Geometry: final body of the model. Coordinates: model frame, mm. Give positions to 0.01 mm unless a question says otherwise; leave off trailing zeros. Write each loop counter-clockwise with the first axis right and the second up, starting at its lowest first coordinate (ties: lowest second). Pieces come first, ordered by that corner, then holes.
```python
from build123d import *

# Parameters (mm, degrees)
SKIZZE2_W                       = 65
SKIZZE2_H                       = 12
AUFSATZ_LINEAR_AUSTRAGEN1_DEPTH = 4
SKIZZE3_R                       = 1.7
SCHNITT_LINEAR_AUSTRAGEN1_DEPTH = 70.241173381
SKIZZE4_R                       = 3.25
SCHNITT_LINEAR_AUSTRAGEN2_DEPTH = 3.2
VERRUNDUNG3_R                   = 1.2


with BuildPart() as part:
    # Skizze2 → Aufsatz-Linear austragen1 (new body)
    with BuildSketch(Plane.XY.offset(18)):
        with Locations((34.289745228, 11.817688499)):
            Rectangle(SKIZZE2_W, SKIZZE2_H)
    extrude(amount=AUFSATZ_LINEAR_AUSTRAGEN1_DEPTH)

    # Skizze3 → Schnitt-Linear austragen1 (cut, through all)
    with BuildSketch(Plane.XY.offset(22)):
        with Locations((21.789745228, 11.817688499)):
            Circle(SKIZZE3_R)
        with Locations((46.789745228, 11.817688499)):
            Circle(SKIZZE3_R)
    extrude(amount=-SCHNITT_LINEAR_AUSTRAGEN1_DEPTH, mode=Mode.SUBTRACT)

    # Skizze4 → Schnitt-Linear austragen2 (cut)
    with BuildSketch(Plane.XY.offset(22)):
        with Locations((21.789745228, 11.817688499)):
            Circle(SKIZZE4_R)
        with Locations((46.789745228, 11.817688499)):
            Circle(SKIZZE4_R)
    extrude(amount=-SCHNITT_LINEAR_AUSTRAGEN2_DEPTH, mode=Mode.SUBTRACT)

    # Verrundung3
    verrundung3_edges = [part.edges().sort_by_distance(p)[0] for p in [
        (1.789745228, 17.817688499, 20),
        (66.789745228, 17.817688499, 20),
        (66.789745228, 5.817688499, 20),
        (1.789745228, 5.817688499, 20),
    ]]
    fillet(verrundung3_edges, radius=VERRUNDUNG3_R)


solid = part.part
```
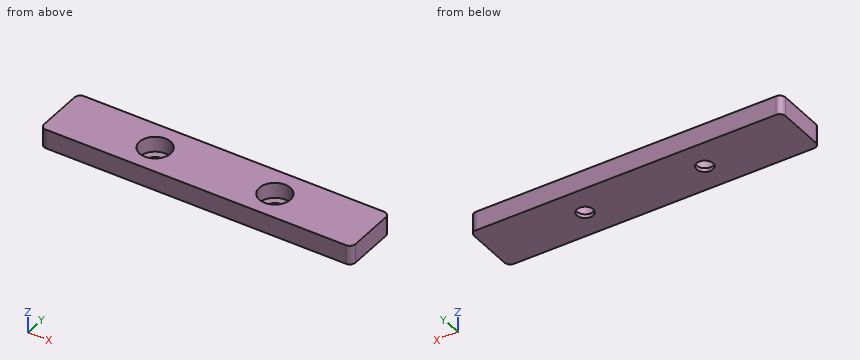
Item 1: Section A-A, the plane y = 10.75. Return the cut outline in (x, z).
Found:
outline: (1.79, 18) - (20.47, 18) - (20.47, 18.8) - (18.72, 18.8) - (18.72, 22) - (1.79, 22) - close; (23.11, 18) - (45.47, 18) - (45.47, 18.8) - (43.72, 18.8) - (43.72, 22) - (24.86, 22) - (24.86, 18.8) - (23.11, 18.8) - close; (48.11, 18) - (66.79, 18) - (66.79, 22) - (49.86, 22) - (49.86, 18.8) - (48.11, 18.8) - close
Item 2: Section C-C, the plane x = 49.5. Return the cut outline in (y, z).
Found:
outline: (5.82, 18) - (17.82, 18) - (17.82, 22) - (13.61, 22) - (13.61, 18.8) - (10.02, 18.8) - (10.02, 22) - (5.82, 22) - close
Item 3: Pin query (flat end, axial travel): pin 1 Ø3 at (x, y) = (46.79, 11.82) entering from -Z. Return the tip coordinate at first contact, or that it passes through.
Found:
pin 1: passes through
Item 4: Section B-B, the plane z = 20.15. Return the cut outline in (x, y).
Found:
outline: (1.79, 7.02) arc R1.2 ccw to (2.99, 5.82) - (65.59, 5.82) arc R1.2 ccw to (66.79, 7.02) - (66.79, 16.62) arc R1.2 ccw to (65.59, 17.82) - (2.99, 17.82) arc R1.2 ccw to (1.79, 16.62) - close; hole circle Ø6.5 at (21.79, 11.82); hole circle Ø6.5 at (46.79, 11.82)
Item 5: Line query: L1, parallel to X at y = 12, z = 18.95; L2, parallel to X at y = 12.75, z = 20.3; L3, parallel to Y at x = 24, z = 20.45. Output: solid intervals per line, ascending.
Found:
L1: x = 1.79 to 18.54, 25.03 to 43.54, 50.03 to 66.79
L2: x = 1.79 to 18.68, 24.9 to 43.68, 49.9 to 66.79
L3: y = 5.82 to 9.43, 14.2 to 17.82
